from build123d import *

# Parameters (mm, degrees)
SKETCH_1_R      = 14.3
EXTRUDE_1_DEPTH = 9


with BuildPart() as part:
    # Sketch 1 → Бобышка-Вытянуть1 (new body)
    with BuildSketch(Plane.XY):
        with BuildLine():
            Line((-55, -108.08739831), (-55, -148.08739831))
            Line((-55, -148.08739831), (-60, -139.427144273))
            ThreePointArc((-60, -139.427144273), (-68.056385746, -80.406003175), (-32.47221146, -32.633971733))
            ThreePointArc((-32.47221146, -32.633971733), (-22.286605842, -20.795527399), (-21.113695467, -5.222486356))
            ThreePointArc((-21.113695467, -5.222486356), (0, 21.75), (21.113695467, -5.222486356))
            ThreePointArc((21.113695467, -5.222486356), (22.286605842, -20.795527399), (32.47221146, -32.633971733))
            ThreePointArc((32.47221146, -32.633971733), (68.056385746, -80.406003175), (60, -139.427144273))
            Line((60, -139.427144273), (55, -148.08739831))
            Line((55, -148.08739831), (55, -108.08739831))
            Line((55, -108.08739831), (57.5, -108.08739831))
            ThreePointArc((57.5, -108.08739831), (0, -52.25), (-57.5, -108.08739831))
            Line((-57.5, -108.08739831), (-55, -108.08739831))
        make_face()
        Circle(SKETCH_1_R, mode=Mode.SUBTRACT)
    extrude(amount=EXTRUDE_1_DEPTH)


solid = part.part
Verification items for the finished model (mm, model axes). A direction names the side the tool comes from. Round coordinates to 2 decimals unless told otherwise and drop trailing zeros. Order: outer loops, then holes, each group sorted by start corner. A loop starts at its lowest first (then second) coordinate and runs counter-clockwise, first axis right, second up.
1. Section check D-D on x = 27.5. Record the cut outline in (y, z), then the cut area to 3 significant figures.
Final values:
outline: (-59.25, 0) - (-28.7, 0) - (-28.7, 9) - (-59.25, 9) - close
area: 275 mm2
2. Section check A-A on y = 0. Record the cut outline in (x, z), then the cut area to 3 significant figures.
Final values:
outline: (-21.75, 0) - (-14.3, 0) - (-14.3, 9) - (-21.75, 9) - close; (14.3, 0) - (21.75, 0) - (21.75, 9) - (14.3, 9) - close
area: 134 mm2
3. Access from +Z, -Z, +X, -X, +Y, -Y to the whole of each face (thin tool, end or side, straight path). Record for faces 1 (the flat face through (-55, -128, 4)), 2 (the cylindrical face through (1.241, -52.263, 4.437)), 3 (the cylindrical face through (-22.373, -21.001, 4.437)).
Final values:
face 1: +Z, -Z, -Y
face 2: +Z, -Z
face 3: +Z, -Z, -X
4. Release check for a two-part mould opening along X. For faces 4 (the flat face through (55, -128, 4)), 5 (the cylindrical face through (-1.86, 14.18, 4.44)), 6 (the flat face through (-57.465, -143.818, 4.437)), 7 (the flat face through (6, -50, 9)) record: +X half, -X half, draft (parallel to the pull), parting line (faces both ways), or undercut.
Final values:
face 4: undercut
face 5: undercut
face 6: -X half
face 7: draft
5. Section check C-C on z = 6.25. Record the cut outline in (x, y), then the cut area to 3 significant figures.
Final values:
outline: (-60, -139.43) - (-55, -148.09) - (-55, -108.09) - (-57.5, -108.09) arc R57.52 cw to (57.5, -108.09) - (55, -108.09) - (55, -148.09) - (60, -139.43) arc R78.74 ccw to (32.47, -32.63) arc R25 cw to (21.11, -5.22) arc R21.75 ccw (long way) to (-21.11, -5.22) arc R25 cw to (-32.47, -32.63) arc R78.74 ccw to start; hole circle Ø28.6 at (0, 0)
area: 6,490 mm2
6. Thickness scan on L1, parallel to Y at x = 0, z = 2.75; L2, parallel to Y at x = 12, z = 7.75; L3, parallel to X at y = 11.5, z = 6. Record the ranges inside material, lowest first.
Final values:
L1: y = -52.25 to -14.3, 14.3 to 21.75
L2: y = -53.52 to -7.78, 7.78 to 18.14
L3: x = -18.46 to -8.5, 8.5 to 18.46
7. Go/stop test with flat-tipped pins: P1, Ø12, axis at x = 34, y = -72.5, coming from the -Z side; P2, Ø4.5, axis at y = -134, z = 3.5, coming from the +X side; P3, Ø1.5, axis at x = -20.5, z = 5.5, coming from the -Y side; P4, Ø0.8, axis at x = -56, z = 5.5, coming from the +Y side. Record where each tip stops, or that it passes through.
Final values:
P1: passes through
P2: stops at x = 63.89
P3: stops at y = -56.32
P4: stops at y = -53.9
8. Section check B-B on x = 0. Record the cut outline in (y, z).
Final values:
outline: (-52.25, 0) - (-14.3, 0) - (-14.3, 9) - (-52.25, 9) - close; (14.3, 0) - (21.75, 0) - (21.75, 9) - (14.3, 9) - close
